Build history of the part. All positions in model axes, mm. A direction names the side the tool comes from. Coordinates: 2 decimals unless noted, no trailing zeros. Write each loop counter-clockwise with the first axis right and the second up, starting at its lowest first coordinate (ties: lowest second). Pieces come first, ordered by that corner, then holes.
from build123d import *

# Parameters (mm, degrees)
EXTRUDE_1_DEPTH     = 7
CUT_EXTRUDE_START   = -5
SKETCH_2_R          = 4
CUT_EXTRUDE_1_DEPTH = 5
SKETCH_3_W          = 29.5
SKETCH_3_H          = 11
EXTRUDE_2_DEPTH     = 8
SKETCH_4_W          = 7.5
SKETCH_4_H          = 10
SKETCH_4_W_2        = 10
EXTRUDE_3_DEPTH     = 7
SKETCH_5_W          = 9
SKETCH_5_H          = 9
CUT_EXTRUDE_2_DEPTH = 2
SKETCH_6_R          = 2.5
CUT_EXTRUDE_3_DEPTH = 2.2
SKETCH_7_R          = 1.6
CUT_EXTRUDE_4_DEPTH = 45.443784717
SKETCH_8_W          = 11.533749137
SKETCH_8_H          = 5
EXTRUDE_4_DEPTH     = 3
CUT_EXTRUDE_5_DEPTH = 3


# Read off the part's stored shape, not the designer's step: 圆顶1, 圆顶2
with BuildPart() as part:
    # 草图1 → 凸台-拉伸1 (new body)
    with BuildSketch(Plane(origin=(0, 0, 0), x_dir=(1, 0, 0), z_dir=(0, 1, 0))):
        with BuildLine():
            Line((0, 0), (29.5, 0))
            Line((29.5, 0), (29.5, -2.5))
            Line((29.5, -2.5), (33.5, -2.5))
            ThreePointArc((33.5, -2.5), (37.5, -6.5), (33.5, -10.5))
            Line((33.5, -10.5), (29.5, -10.5))
            Line((29.5, -10.5), (29.5, -13))
            Line((29.5, -13), (0, -13))
            Line((0, -13), (0, -10.5))
            Line((0, -10.5), (-4, -10.5))
            ThreePointArc((-4, -10.5), (-8, -6.5), (-4, -2.5))
            Line((-4, -2.5), (0, -2.5))
            Line((0, -2.5), (0, 0))
        make_face()
    extrude(amount=EXTRUDE_1_DEPTH)

    # 草图2 → 切除-拉伸1 (cut)
    with BuildSketch(Plane(origin=(0, 7, 0), x_dir=(1, 0, 0), z_dir=(0, 1, 0)).offset(CUT_EXTRUDE_START)):
        with Locations((-4, -6.5)):
            Circle(SKETCH_2_R)
        with Locations((33.5, -6.5)):
            Circle(SKETCH_2_R)
    extrude(amount=CUT_EXTRUDE_1_DEPTH, mode=Mode.SUBTRACT)

    # 草图3 → 凸台-拉伸2 (add)
    with BuildSketch(Plane(origin=(0, 7, 0), x_dir=(1, 0, 0), z_dir=(0, 1, 0))):
        with Locations((14.75, -6.5)):
            Rectangle(SKETCH_3_W, SKETCH_3_H)
    extrude(amount=EXTRUDE_2_DEPTH)

    # 草图4 → 凸台-拉伸3 (add)
    with BuildSketch(Plane(origin=(0, 15, 0), x_dir=(1, 0, 0), z_dir=(0, 1, 0))):
        with Locations((25.25, -6.5)):
            Rectangle(SKETCH_4_W, SKETCH_4_H)
        with Locations((5.5, -6.5)):
            Rectangle(SKETCH_4_W_2, SKETCH_4_H)
    extrude(amount=EXTRUDE_3_DEPTH)

    # 草图5 → 切除-拉伸2 (cut)
    with BuildSketch(Plane(origin=(0, 22, 0), x_dir=(1, 0, 0), z_dir=(0, 1, 0))):
        with Locations((5.5, -6.5)):
            Rectangle(SKETCH_5_W, SKETCH_5_H)
    extrude(amount=-CUT_EXTRUDE_2_DEPTH, mode=Mode.SUBTRACT)

    # 草图6 → 切除-拉伸3 (cut)
    with BuildSketch(Plane(origin=(0, 22, 0), x_dir=(1, 0, 0), z_dir=(0, 1, 0))):
        with Locations(Location((25.25, -6.5, 0), (0, 0, 270))):
            Circle(SKETCH_6_R)
        with Locations(Location((4.253331237, -6.5, 0), (0, 0, 270))):
            Circle(SKETCH_6_R)
    extrude(amount=-CUT_EXTRUDE_3_DEPTH, mode=Mode.SUBTRACT)

    # 圆顶1 outline → 圆顶1 (revolve)
    with BuildSketch(Plane(origin=(4.253331237, 0, 6.5), x_dir=(1, 0, 0), z_dir=(0, 0, 1))):
        with BuildLine():
            Line((0, 19.8), (2.500000001, 19.799999998))
            ThreePointArc((2.500000001, 19.799999998), (1.60078106, 21.238476323), (0, 21.8))
            Line((0, 21.8), (0, 19.8))
        make_face()
    revolve(axis=Axis((4.253331237, 0, 6.5), (0, 1, 0)))

    # 圆顶2 outline → 圆顶2 (revolve)
    with BuildSketch(Plane(origin=(25.25, 0, 6.5), x_dir=(1, 0, 0), z_dir=(0, 0, 1))):
        with BuildLine():
            Line((0, 19.8), (2.500000001, 19.799999997))
            ThreePointArc((2.500000001, 19.799999997), (1.60078106, 21.238476323), (0, 21.8))
            Line((0, 21.8), (0, 19.8))
        make_face()
    revolve(axis=Axis((25.25, 0, 6.5), (0, 1, 0)))

    # 草图7 → 切除-拉伸4 (cut, through all)
    with BuildSketch(Plane(origin=(0, 2, 0), x_dir=(1, 0, 0), z_dir=(0, 1, 0))):
        with Locations(Location((-4, -6.5, 0), (0, 0, 270))):
            Circle(SKETCH_7_R)
        with Locations(Location((33.5, -6.5, 0), (0, 0, 270))):
            Circle(SKETCH_7_R)
    extrude(amount=-CUT_EXTRUDE_4_DEPTH, mode=Mode.SUBTRACT)

    # 草图8 → 凸台-拉伸4 (add)
    with BuildSketch(Plane.XY.offset(13)):
        with Locations((14.355989937, 2.5)):
            Rectangle(SKETCH_8_W, SKETCH_8_H)
    extrude(amount=EXTRUDE_4_DEPTH)

    # 草图10 → 切除-拉伸5 (cut)
    with BuildSketch(Plane.XZ):
        Polygon((8.589115368, 16), (8.589115368, 12), (1, 12), (1, 1), (28.5, 1), (28.5, 12), (20.122864505, 12), (20.122864505, 16), align=None)
    extrude(amount=-CUT_EXTRUDE_5_DEPTH, mode=Mode.SUBTRACT)


solid = part.part
(1) Slice it at C-C, the plane z = 9.75. List the corners of the cut face in (x, y).
(2) 3-axis set-ups, long thin cutter, end or side, ignore diameter. For faces 1 (the flat face through (5, 18, 1.5)), 2 (the flat face through (5, 18, 11.5)), 3 (the flat face through (24, 1, 12)), 4 (the flat face through (-2, 3, 2.5)): which of +Z, -Z, +X, -X, +Y, -Y reach the whole face in a straight line?
(3) Probe L1, parallel to X at y = 0.65, z = 6.5; L2, parallel to X at y = 19, z = 7.5; L3, parallel to Z at x = 2, y = 2.5. List the from-to ranges inside material, lowest first.
(4) Slice it at A-A, the plane y = 16. List the corners of the cut face in (x, z).
(5) Slice it at D-D, the plane y = 6. List the corners of the cut face in (x, z), and give its area (3 significant figures).
(6) Slice it at B-B, the plane x = 19. List the corners of the cut face in (y, z).
(7) Flat gauge pins, fed straight in: P1, Ø7.5, axis at x = 17, z = 9, coming from the -Y side; P2, Ø3.5, axis at x = 25, y = 19, coming from the -Z side; P3, Ø1, axis at y = 8, z = 4, coming from the +X side. Where does each tip first touch, or does it go through?
(8) Two-plate mould, pull along Z, no slides. Class faces 5 (the flat face through (15, 15, 6)), 6 (the flat face through (10, 21, 7)), 7 (the flat face through (-2, 3, 10.5)): pulls with the +Z half, pulls with the -Z half, needs draft (parallel to the pull), parting line crosses it, or undercut.
Results:
1. outline: (-6.33, 0) - (1, 0) - (1, 3) - (28.5, 3) - (28.5, 0) - (35.83, 0) - (35.83, 2) - (31.17, 2) - (31.17, 7) - (29.5, 7) - (29.5, 15) - (29, 15) - (29, 22) - (21.5, 22) - (21.5, 15) - (10.5, 15) - (10.5, 22) - (10, 22) - (10, 20) - (1, 20) - (1, 22) - (0.5, 22) - (0.5, 15) - (0, 15) - (0, 7) - (-1.67, 7) - (-1.67, 2) - (-6.33, 2) - close
2. face 1: -Z, +X, -X, +Y
2. face 2: +Z, +X, -X, +Y
2. face 3: -Y
2. face 4: -Z, -X, +Y, -Y
3. L1: x = -8 to -5.6, -2.4 to 1, 28.5 to 31.9, 35.1 to 37.5
3. L2: x = 0.5 to 10.5, 21.5 to 29
3. L3: z = 0 to 1, 12 to 13
4. outline: (0.5, 1.5) - (10.5, 1.5) - (10.5, 11.5) - (0.5, 11.5) - close; (21.5, 1.5) - (29, 1.5) - (29, 11.5) - (21.5, 11.5) - close
5. outline: (-4, 2.5) - (0, 2.5) - (0, 0) - (29.5, 0) - (29.5, 2.5) - (33.5, 2.5) arc R4 cw to (33.5, 10.5) - (29.5, 10.5) - (29.5, 13) - (0, 13) - (0, 10.5) - (-4, 10.5) arc R4 cw to start
5. area: 397 mm2
6. outline: (0, 0) - (7, 0) - (7, 1) - (15, 1) - (15, 12) - (7, 12) - (7, 13) - (5, 13) - (5, 16) - (3, 16) - (3, 1) - (0, 1) - close
7. P1: stops at y = 3
7. P2: stops at z = 1.5
7. P3: stops at x = 29.5
8. face 5: needs draft
8. face 6: undercut
8. face 7: pulls with the +Z half
